Here's how the part is built. I have some questions about the finished solid (model axes, mm). Round coordinates to 2 decimals unless told otherwise and drop trailing zeros. Loops run counter-clockwise (first coordinate to the right, second up) from the corner with the lowest first, then second, coordinate; pieces in that order, holes last. Notation, with made-up numbers: M -15,60.25 L 3,60.25 A20 ccw 3,81.25 Z; hole C -37,74.5 d1. An arc over 180 degrees is marked long. Answer as CSV lines item,"result".
```python
from build123d import *

# Parameters (mm, degrees)
F0_W     = 40
F0_H     = 40
F1_DEPTH = 2
F2_W     = 2
F2_H     = 34
F3_DEPTH = 20
F4_W     = 18
F4_H     = 30
F5_DEPTH = 40.001
F6_W     = 2
F6_H     = 6
F7_DEPTH = 2


# Not quite as in the source:
# - the program builds the solid bodies; features that only make, move or delete a surface that nothing else refers to are left out


with BuildPart() as f1:
    # F0 (on Front) → F1 (new body)
    with BuildSketch(Plane.XZ):
        with Locations((-31.0945767164, 25.4016729393)):
            Rectangle(F0_W, F0_H)
    extrude(amount=F1_DEPTH)

    # F2 (on face) → F3 (join)
    with BuildSketch(Plane.XZ.offset(2)):
        with Locations((-50.0945767164, 28.4016729393)):
            Rectangle(F2_W, F2_H)
    extrude(amount=F3_DEPTH)

    # F4 (on face) → F5 (cut, through all)
    with BuildSketch(Plane(origin=(-51.0945767164, 0, 0), x_dir=(0, -1, 0), z_dir=(-1, 0, 0))):
        with Locations((11, 28.4016729393)):
            Rectangle(F4_W, F4_H)
    extrude(amount=-F5_DEPTH, mode=Mode.SUBTRACT)

    # F6 (on face) → F7 (cut)
    with BuildSketch(Plane(origin=(-51.0945767164, 0, 0), x_dir=(0, -1, 0), z_dir=(-1, 0, 0))):
        with Locations((1, 8.4016729393)):
            Rectangle(F6_W, F6_H)
    extrude(amount=-F7_DEPTH, mode=Mode.SUBTRACT)


solid = f1.part
```
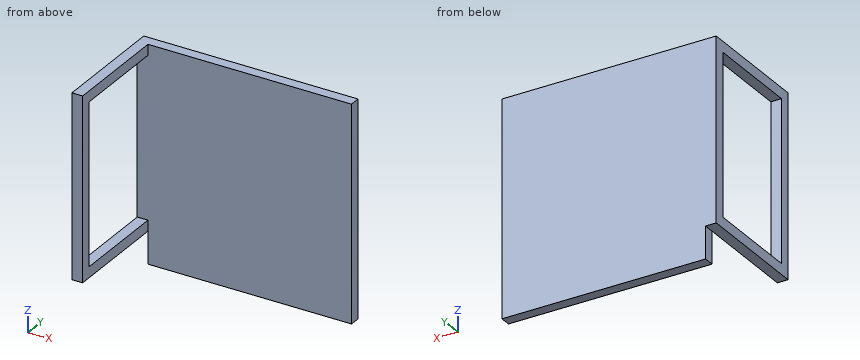
1. If I drill on line 1 (Y direction, x = -46, z = 37.5), over which ranges is the centre line in solid material (lowest first)? Write a range as [from, to].
Evaluation:
line 1,"y = [-2, 0]"
2. I want a section at A-A, the plane y = -17.5. Please give me the cut outline in (x, z).
Evaluation:
outline,"M -51.09,11.4 L -49.09,11.4 L -49.09,13.4 L -51.09,13.4 Z; M -51.09,43.4 L -49.09,43.4 L -49.09,45.4 L -51.09,45.4 Z"
3. I want a section at B-B, the plane z = 27.5. Please give me the cut outline in (x, y), and give its area (3 significant figures).
Evaluation:
outline,"M -51.09,-22 L -49.09,-22 L -49.09,-20 L -51.09,-20 Z; M -51.09,-2 L -11.09,-2 L -11.09,0 L -51.09,0 Z"
area,"84.0 mm²"
4. I want a section at C-C, the plane x = -46.5. Please give me the cut outline in (y, z).
Evaluation:
outline,"M -2,5.4 L 0,5.4 L 0,45.4 L -2,45.4 Z"
5. For P1, Ø3, axis at x = -42, y = -5, coming from the -Z side; P2, Ø2, axis at x = -40, z = 22.5, coming from the -Y side; P3, Ø6, axis at y = -17.5, z = 38.5, coming from the +X side; P4, Ø1, axis at y = -1, z = 8, coming from the -X side, each with a flat end and sliding along its axis, tell me the tip position at first contact or that it passes through.
Evaluation:
P1,"passes through"
P2,"stops at y = -2"
P3,"stops at x = -49.09"
P4,"stops at x = -49.09"
